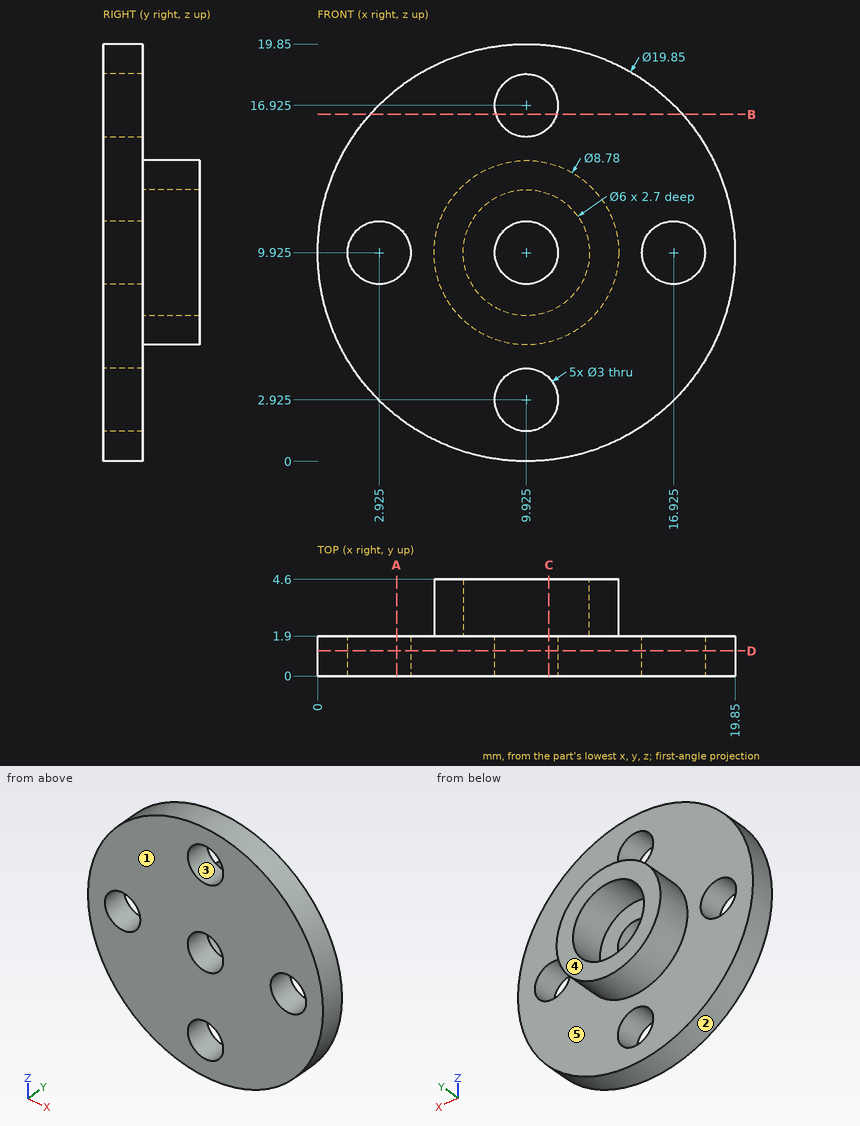
Here's the drawing with two shaded views (mm, measured from the low corner). I have some questions. A direction names the side the tool comes from. Give positions to 0.01 mm unless a question says otherwise; leave off trailing zeros. Loops run counter-clockwise (first coordinate to the right, second up) from the corner with the lowest first, then second, coordinate; pieces in that order, holes last. Notation, with made-up numbers: (17, 59) - (39, 59) arc R24 cw to (39, 83) - close; hole circle Ø1 at (10.25, 24.5). An arc over 180 degrees is marked (long way). Answer in a Markdown table with one row per item. Add a question column.
Q1. If we section it at D-D (y = 1.2): List the corners of the cut face in (x, z) for me (3 decimals).
Q2. If we section it at B-B (z = 16.5): List the corners of the cut face in (x, y) for me.
Q3. Please list where these lines run through material, in increasing order: L1, parallel to Y at x = 15.5, z = 3; L2, parallel to X at y = 4.3, z = 11; L3, parallel to X at y = 2.15, z = 10. Write a range as from..to.
Q4. We'd pull the mould along Z, two halves only. Please class the marked faces 1, 2 and 3: +Z half, -Z half, draft (parallel to the pull), parting line (faces both ways), or undercut.
Q5. If we section it at C-C (x = 11): List the corners of the cut face in (y, z) for me.
Q6. For pin 1 (1 mm diameter, centred on x = 6.5, z = 5.5, fed in from +Y); pin 2 (1.5 mm diameter, centred on x = 17.5, y = 1, fed in from +Z), each with a flat end and sliding along its axis, tell me the tip position at first contact or that it passes through.
Q7. Which directions (+Z, -Z, +X, -X, +Y, -Y) give clear straight access to the entire face, cutting with the end or side of a thin tool? Please do the marked faces 4 and 5.
Q8. If we section it at A-A (x = 3.75): List the corners of the cut face in (y, z) for me.
The answers:
| question | item | result |
|---|---|---|
| 1 | outline | circle Ø19.85 at (9.925, 9.925); hole circle Ø3 at (2.925, 9.925); hole circle Ø3 at (9.925, 2.925); hole circle Ø3 at (9.925, 9.925); hole circle Ø3 at (9.925, 16.925); hole circle Ø3 at (16.925, 9.925) |
| 2 | outline | (2.49, 0) - (8.49, 0) - (8.49, 1.9) - (2.49, 1.9) - close; (11.36, 0) - (17.36, 0) - (17.36, 1.9) - (11.36, 1.9) - close |
| 3 | L1 | y = 0..1.9 |
| 3 | L2 | x = 5.67..7.12, 12.73..14.18 |
| 3 | L3 | x = 5.54..6.93, 12.92..14.31 |
| 4 | face 1 | draft |
| 4 | face 2 | parting line |
| 4 | face 3 | undercut |
| 5 | outline | (0, 0.06) - (1.9, 0.06) - (1.9, 1.88) - (0, 1.88) - close; (0, 3.97) - (1.9, 3.97) - (1.9, 5.67) - (4.6, 5.67) - (4.6, 7.12) - (1.9, 7.12) - (1.9, 8.88) - (0, 8.88) - close; (0, 10.97) - (1.9, 10.97) - (1.9, 12.73) - (4.6, 12.73) - (4.6, 14.18) - (1.9, 14.18) - (1.9, 15.88) - (0, 15.88) - close; (0, 17.97) - (1.9, 17.97) - (1.9, 19.79) - (0, 19.79) - close |
| 6 | pin 1 | stops at y = 1.9 |
| 6 | pin 2 | stops at z = 17.13 |
| 7 | face 4 | +Z, -Z, +X, -X, +Y |
| 7 | face 5 | +Y |
| 8 | outline | (0, 2.15) - (1.9, 2.15) - (1.9, 8.67) - (0, 8.67) - close; (0, 11.18) - (1.9, 11.18) - (1.9, 17.7) - (0, 17.7) - close |
